Check sheet for the modelled part. Datum: model origin and axes. Units: mm. A direction names the side the tool comes from. Coordinates: 2 decimals unless noted, no trailing zeros. Order: outer loops, then holes, each group sorted by start corner. A loop starts at its lowest first (then second) coordinate and runs counter-clockwise, first axis right, second up.
1. Thickness scan on line 1 (X direction, y = -1.75, z = 21); line 2 (X direction, y = -3.7, z = 15); line 3 (Z direction, x = 47, y = 5.5). Record the ranges inside material, lowest first.
2. Cross-section at A-A (z = 6.2). Enter the section's corners in (x, y), then the cut area to 3 significant figures.
3. Cross-section at D-D (y = 7.75). Enter the section's corners in (x, z).
4. Set-up check for faces 4 (the cylindrical face through (-16.865, 1.318, 1.479)), 5 (the flat face through (6, -1.107, 13)), 6 (the cylindrical face through (50.73, -3.61, 21.86)): record each of +Z, -Z, +X, -X, +Y, -Y from which the full face is reachable in a straight line by a thin tool's end or side.
5. Gauge pin test, flat ends, axial feed: pin 1 Ø4.5 at (x, z) = (-31.65, 6.2) entering from +Y; pin 2 Ø4 at (x, y) = (0, 7) entering from +Z; pin 3 Ø1.3 at (x, z) = (49, 14) entering from -Y; pin 4 Ø2.5 at (x, y) = (-18.25, 1.89) entering from -Z. Record the tip position at first contact, or that the pin passes through.
6. Cross-section at B-B (x = 21). Enter the section's corners in (y, z), then the cut area to 3 significant figures.
7. Cross-section at C-C (x = 44). Enter the section's corners in (y, z), then the cut area to 3 significant figures.
8. Draft check along X on faces 1 (the flat face through (-38.251, -2, 12)), 2 (the flat face through (-34, -3.107, 21)), 3 (the flat face through (48.19, 5.85, 1.48)). Enter one of: released by +X, released by -X, zero draft, split by the parting line, or undercut.
```python
from build123d import *

# Parameters (mm, degrees)
SKETCH1_R           = 1.5
BOSS_EXTRUDE1_DEPTH = 3
SKETCH1_3_W         = 89.4
SKETCH1_3_H         = 3
BOSS_EXTRUDE2_DEPTH = 24
CUT_EXTRUDE1_REACH  = 5
SKETCH3_R           = 1.5
SKETCH3_R_2         = 1.75
CUT_EXTRUDE2_START  = -3
SKETCH3_5_R         = 2.25
SKETCH3_5_R_2       = 1.5
CUT_EXTRUDE2_DEPTH  = 1


with BuildPart() as part:
    # Sketch1 → Boss-Extrude1 (new body)
    with BuildSketch(Plane.XY):
        Polygon((-32.2510699, 8.892599614), (-38.2510699, 2.892599614), (-38.2510699, -1.107400386), (51.1489301, -1.107400386), (51.1489301, 2.892599614), (45.1489301, 8.892599614), align=None)
        with Locations((-18.2510699, 1.892599614)):
            Circle(SKETCH1_R, mode=Mode.SUBTRACT)
        with Locations((31.1489301, 1.892599614)):
            Circle(SKETCH1_R, mode=Mode.SUBTRACT)
    extrude(amount=BOSS_EXTRUDE1_DEPTH)

    # Sketch1<3> → Boss-Extrude2 (add)
    with BuildSketch(Plane.XY):
        with Locations((6.4489301, -2.607400386)):
            Rectangle(SKETCH1_3_W, SKETCH1_3_H)
    extrude(amount=BOSS_EXTRUDE2_DEPTH)

    # Sketch3 → Cut-Extrude1 (cut, up to next)
    with BuildSketch(Plane(origin=(0, -1.107400386, 0), x_dir=(1, 0, 0), z_dir=(0, 1, 0)), mode=Mode.PRIVATE) as cut_extrude1_sk1:
        with Locations((48.6489301, -15)):
            Circle(SKETCH3_R)
    cut_extrude1_tool1 = extrude(cut_extrude1_sk1.sketch, amount=-CUT_EXTRUDE1_REACH, mode=Mode.PRIVATE) & part.part
    add(cut_extrude1_tool1.solids().sort_by_distance((48.64893, -1.1074, 15))[0], mode=Mode.SUBTRACT)
    # Sketch3 → Cut-Extrude1 (cut, up to next)
    with BuildSketch(Plane(origin=(0, -1.107400386, 0), x_dir=(1, 0, 0), z_dir=(0, 1, 0)), mode=Mode.PRIVATE) as cut_extrude1_sk2:
        with Locations((48.6489301, -21)):
            Circle(SKETCH3_R)
    cut_extrude1_tool2 = extrude(cut_extrude1_sk2.sketch, amount=-CUT_EXTRUDE1_REACH, mode=Mode.PRIVATE) & part.part
    add(cut_extrude1_tool2.solids().sort_by_distance((48.64893, -1.1074, 21))[0], mode=Mode.SUBTRACT)
    # Sketch3 → Cut-Extrude1 (cut, up to next)
    with BuildSketch(Plane(origin=(0, -1.107400386, 0), x_dir=(1, 0, 0), z_dir=(0, 1, 0)), mode=Mode.PRIVATE) as cut_extrude1_sk3:
        with Locations((-35.7510699, -15)):
            Circle(SKETCH3_R)
    cut_extrude1_tool3 = extrude(cut_extrude1_sk3.sketch, amount=-CUT_EXTRUDE1_REACH, mode=Mode.PRIVATE) & part.part
    add(cut_extrude1_tool3.solids().sort_by_distance((-35.75107, -1.1074, 15))[0], mode=Mode.SUBTRACT)
    # Sketch3 → Cut-Extrude1 (cut, up to next)
    with BuildSketch(Plane(origin=(0, -1.107400386, 0), x_dir=(1, 0, 0), z_dir=(0, 1, 0)), mode=Mode.PRIVATE) as cut_extrude1_sk4:
        with Locations((-35.7510699, -21)):
            Circle(SKETCH3_R)
    cut_extrude1_tool4 = extrude(cut_extrude1_sk4.sketch, amount=-CUT_EXTRUDE1_REACH, mode=Mode.PRIVATE) & part.part
    add(cut_extrude1_tool4.solids().sort_by_distance((-35.75107, -1.1074, 21))[0], mode=Mode.SUBTRACT)
    # Sketch3 → Cut-Extrude1 (cut, up to next)
    with BuildSketch(Plane(origin=(0, -1.107400386, 0), x_dir=(1, 0, 0), z_dir=(0, 1, 0)), mode=Mode.PRIVATE) as cut_extrude1_sk5:
        with Locations((44.5489301, -6.2)):
            Circle(SKETCH3_R_2)
    cut_extrude1_tool5 = extrude(cut_extrude1_sk5.sketch, amount=-CUT_EXTRUDE1_REACH, mode=Mode.PRIVATE) & part.part
    add(cut_extrude1_tool5.solids().sort_by_distance((44.54893, -1.1074, 6.2))[0], mode=Mode.SUBTRACT)
    # Sketch3 → Cut-Extrude1 (cut, up to next)
    with BuildSketch(Plane(origin=(0, -1.107400386, 0), x_dir=(1, 0, 0), z_dir=(0, 1, 0)), mode=Mode.PRIVATE) as cut_extrude1_sk6:
        with Locations((-31.6510699, -6.2)):
            Circle(SKETCH3_R_2)
    cut_extrude1_tool6 = extrude(cut_extrude1_sk6.sketch, amount=-CUT_EXTRUDE1_REACH, mode=Mode.PRIVATE) & part.part
    add(cut_extrude1_tool6.solids().sort_by_distance((-31.65107, -1.1074, 6.2))[0], mode=Mode.SUBTRACT)

    # Sketch3<5> → Cut-Extrude2 (cut)
    with BuildSketch(Plane(origin=(0, -1.107400386, 0), x_dir=(1, 0, 0), z_dir=(0, 1, 0)).offset(CUT_EXTRUDE2_START)):
        with Locations((-35.7510699, -15)):
            Circle(SKETCH3_5_R)
        with Locations((-35.7510699, -15)):
            Circle(SKETCH3_5_R_2, mode=Mode.SUBTRACT)
        with Locations((-35.7510699, -21)):
            Circle(SKETCH3_5_R)
        with Locations((-35.7510699, -21)):
            Circle(SKETCH3_5_R_2, mode=Mode.SUBTRACT)
        with Locations((48.6489301, -15)):
            Circle(SKETCH3_5_R)
        with Locations((48.6489301, -21)):
            Circle(SKETCH3_5_R)
    extrude(amount=CUT_EXTRUDE2_DEPTH, mode=Mode.SUBTRACT)


solid = part.part
```
Data:
1. line 1: x = -38.25 to -37.25, -34.25 to 47.15, 50.15 to 51.15
1. line 2: x = -38.25 to -38, -33.5 to 46.4, 50.9 to 51.15
1. line 3: z = 0 to 3
2. outline: (-38.25, -4.11) - (-33.4, -4.11) - (-33.4, -1.11) - (-38.25, -1.11) - close; (-29.9, -4.11) - (42.8, -4.11) - (42.8, -1.11) - (-29.9, -1.11) - close; (46.3, -4.11) - (51.15, -4.11) - (51.15, -1.11) - (46.3, -1.11) - close
2. area: 247 mm2
3. outline: (-33.39, 0) - (46.29, 0) - (46.29, 3) - (-33.39, 3) - close
4. face 4: +Z, -Z
4. face 5: +Z, +X, -X, +Y
4. face 6: -Y
5. pin 1: stops at y = -1.11
5. pin 2: stops at z = 3
5. pin 3: stops at y = -3.11
5. pin 4: passes through
6. outline: (-4.11, 0) - (8.89, 0) - (8.89, 3) - (-1.11, 3) - (-1.11, 24) - (-4.11, 24) - close
6. area: 102 mm2
7. outline: (-4.11, 0) - (8.89, 0) - (8.89, 3) - (-1.11, 3) - (-1.11, 4.54) - (-4.11, 4.54) - close; (-4.11, 7.86) - (-1.11, 7.86) - (-1.11, 24) - (-4.11, 24) - close
7. area: 92.0 mm2
8. face 1: released by -X
8. face 2: undercut
8. face 3: released by +X
